from build123d import *

# Parameters (mm, degrees)
REVOLVE1_ANGLE           = 180
SKETCH2_R                = 11.607478401
CUT_EXTRUDE1_DEPTH       = 30
REVOLVE3_ANGLE           = 20
REVOLVE3_OTHER_WAY_ANGLE = 20
SKETCH6_W                = 87.695776886
SKETCH6_H                = 110.7877302
CUT_EXTRUDE2_DEPTH       = 30


with BuildPart() as part:
    # Sketch1 → Revolve1 (revolve)
    with BuildSketch(Plane.XY):
        with BuildLine():
            Line((37.03427234, 1.564642505), (18.431130492, 35.41414573))
            add(Edge.make_bspline(
                [(18.431130492, 35.41414573), (14.894772629, 62.905623644), (37.03427234, 76.73235426)],
                knots=[0, 0, 0, 1, 1, 1], degree=2))
            Line((37.03427234, 76.73235426), (37.03427234, 57.257883484))
            ThreePointArc((37.03427234, 57.257883484), (25.426793939, 45.650405083), (37.03427234, 34.042926682))
            Line((37.03427234, 34.042926682), (37.03427234, 1.564642505))
        make_face()
    revolve(axis=Axis((37.03427234, 57.257883484, 0), (0, 1, 0)), revolution_arc=REVOLVE1_ANGLE)

    # Sketch2 → Cut-Extrude1 (cut)
    with BuildSketch(Plane(origin=(0, 0, 0), x_dir=(-1, 0, 0), z_dir=(0, 0, -1))):
        with Locations((-37.03427234, 45.650405083)):
            Circle(SKETCH2_R)
    extrude(amount=-CUT_EXTRUDE1_DEPTH, mode=Mode.SUBTRACT)

    # Sketch3 → Revolve3 (revolve)
    with BuildSketch(Plane(origin=(0, 0, 0), x_dir=(-1, 0, 0), z_dir=(0, 0, -1))):
        with BuildLine():
            Line((-55.774902941, 35.7486794), (-45.306584566, 16.700962649))
            add(Edge.make_bspline(
                [(-45.306584566, 16.700962649), (-54.069804725, 17.26279972), (-62.206909853, 15.470822713)],
                knots=[0, 0, 0, 0.385925107, 0.385925107, 0.385925107], degree=2))
            add(Edge.make_bspline(
                [(-55.774902941, 35.7486794), (-63.0996884, 25.437145822), (-62.206909853, 15.470822713)],
                knots=[0, 0, 0, 0.565089792, 0.565089792, 0.565089792], degree=2))
        make_face()
        with BuildLine():
            Line((-18.293641739, 35.7486794), (-28.761960114, 16.700962649))
            add(Edge.make_bspline(
                [(-28.761960114, 16.700962649), (-19.998739955, 17.26279972), (-11.861634828, 15.470822713)],
                knots=[0, 0, 0, 0.385925107, 0.385925107, 0.385925107], degree=2))
            add(Edge.make_bspline(
                [(-18.293641739, 35.7486794), (-10.96885628, 25.437145822), (-11.861634828, 15.470822713)],
                knots=[0, 0, 0, 0.565089792, 0.565089792, 0.565089792], degree=2))
        make_face()
    revolve(axis=Axis((37.03427234, 76.73235426, 0), (0, -1, 0)), revolution_arc=REVOLVE3_ANGLE)

    # Sketch3 → Revolve3 other way (revolve)
    with BuildSketch(Plane(origin=(0, 0, 0), x_dir=(-1, 0, 0), z_dir=(0, 0, -1))):
        with BuildLine():
            Line((-55.774902941, 35.7486794), (-45.306584566, 16.700962649))
            add(Edge.make_bspline(
                [(-45.306584566, 16.700962649), (-54.069804725, 17.26279972), (-62.206909853, 15.470822713)],
                knots=[0, 0, 0, 0.385925107, 0.385925107, 0.385925107], degree=2))
            add(Edge.make_bspline(
                [(-55.774902941, 35.7486794), (-63.0996884, 25.437145822), (-62.206909853, 15.470822713)],
                knots=[0, 0, 0, 0.565089792, 0.565089792, 0.565089792], degree=2))
        make_face()
        with BuildLine():
            Line((-18.293641739, 35.7486794), (-28.761960114, 16.700962649))
            add(Edge.make_bspline(
                [(-28.761960114, 16.700962649), (-19.998739955, 17.26279972), (-11.861634828, 15.470822713)],
                knots=[0, 0, 0, 0.385925107, 0.385925107, 0.385925107], degree=2))
            add(Edge.make_bspline(
                [(-18.293641739, 35.7486794), (-10.96885628, 25.437145822), (-11.861634828, 15.470822713)],
                knots=[0, 0, 0, 0.565089792, 0.565089792, 0.565089792], degree=2))
        make_face()
    revolve(axis=Axis((37.03427234, 76.73235426, 0), (0, 1, 0)), revolution_arc=REVOLVE3_OTHER_WAY_ANGLE)

    # Sketch6 → Cut-Extrude2 (cut)
    with BuildSketch(Plane(origin=(0, 0, 0), x_dir=(-1, 0, 0), z_dir=(0, 0, -1))):
        with Locations((-37.762446628, 42.00670517)):
            Rectangle(SKETCH6_W, SKETCH6_H)
    extrude(amount=CUT_EXTRUDE2_DEPTH, mode=Mode.SUBTRACT)


solid = part.part
Verification items for the finished model (mm, model axes). A direction names the side the tool comes from. Give positions to 0.01 mm unless a question says otherwise; leave off trailing zeros.
(1) Access from +Z, -Z, +X, -X, +Y, -Y to the whole of each face (thin tool, end or side, straight path). Record for faces 3 (the face through (19.142, 23.499, 6.512)), 4 (the face through (39.55, 34.32, 8.8)).
(2) Mould release check, pull along X, two halves, no side actions. Record for faces 1 (the face through (36.872, 14.965, 7.363)), 2 (the face through (37, 31, 0)): +X half, -X half, draft (parallel to the pull), parting line (faces both ways), or undercut.
(3) Cross-section at A-A (z = 7.25). State how many separate pieces and enclosed holes the cut face has, plus the area to 3 significant figures.
(4) Material ranges on line 1 (X direction, y = 37, z = 10); line 2 (Y direction, x = 29.5, z = 12.25); line 3 (Y direction, x = 30, z = 2.5), recorded low to high.
(5) Gauge pin test, flat ends, axial feed: pin 1 (2 mm diameter, centred on y = 25, z = 4.5, fed in from -X); pin 2 (5 mm diameter, centred on x = 36, y = 64.5, fed in from +Z); pin 3 (10 mm diameter, centred on x = 24.5, y = 66, fed in from +Z); pin 4 (5 mm diameter, centred on x = 23.5, y = 22.5, fed in from -Z). Record the tip position at first contact, or that the pin passes through.
Worked out:
1. face 3: +Z, -Y
1. face 4: +Z, -Z
2. face 1: undercut
2. face 2: draft
3. separate pieces: 3
3. enclosed holes: 1
3. area: 1,130 mm2
4. line 1: x = 21.13 to 29.29, 44.77 to 52.94
4. line 2: y = 27.73 to 36.82, 54.48 to 62.16
4. line 3: y = 15.15 to 36.42, 54.88 to 71
5. pin 1: stops at x = 12.95
5. pin 2: stops at z = 14.44
5. pin 3: stops at z = 11
5. pin 4: stops at z = 0
